from build123d import *

# Parameters (mm, degrees)
BOSS_EXTRUDE1_DEPTH = 4.7625


with BuildPart() as part:
    # Sketch2 → Boss-Extrude1 (new body)
    with BuildSketch(Plane.XY):
        with BuildLine():
            Line((-23, -45.048102255), (-1, -45.048102255))
            ThreePointArc((-1, -45.048102255), (-0.292893219, -45.340995473), (0, -46.048102255))
            Line((0, -46.048102255), (0, -57.748102255))
            Line((0, -57.748102255), (4.7625, -57.748102255))
            Line((4.7625, -57.748102255), (4.7625, -46.048102255))
            ThreePointArc((4.7625, -46.048102255), (5.055393219, -45.340995473), (5.7625, -45.048102255))
            Line((5.7625, -45.048102255), (11.7625, -45.048102255))
            ThreePointArc((11.7625, -45.048102255), (12.469606781, -45.340995473), (12.7625, -46.048102255))
            Line((12.7625, -46.048102255), (12.7625, -69.765561421))
            ThreePointArc((12.7625, -69.765561421), (12.805346982, -70.055144052), (12.9302162, -70.319911199))
            Line((12.9302162, -70.319911199), (68, -153))
            Line((68, -153), (68, -156.7625))
            ThreePointArc((68, -156.7625), (67.707106781, -157.469606781), (67, -157.7625))
            Line((67, -157.7625), (61, -157.7625))
            ThreePointArc((61, -157.7625), (60.292893219, -157.469606781), (60, -156.7625))
            Line((60, -156.7625), (60, -153))
            Line((60, -153), (45.481563848, -153))
            Line((45.481563848, -153), (45.481563848, -156.7625))
            ThreePointArc((45.481563848, -156.7625), (45.188670629, -157.469606781), (44.481563848, -157.7625))
            Line((44.481563848, -157.7625), (38.481563848, -157.7625))
            ThreePointArc((38.481563848, -157.7625), (37.774457067, -157.469606781), (37.481563848, -156.7625))
            Line((37.481563848, -156.7625), (37.481563848, -153))
            Line((37.481563848, -153), (13.059329161, -116.333203921))
            ThreePointArc((13.059329161, -116.333203921), (12.699088908, -116.005978468), (12.227045361, -115.8875537))
            Line((12.227045361, -115.8875537), (-36.227045361, -115.8875537))
            ThreePointArc((-36.227045361, -115.8875537), (-36.699088908, -116.005978468), (-37.059329161, -116.333203921))
            Line((-37.059329161, -116.333203921), (-61.481563848, -153))
            Line((-61.481563848, -153), (-61.481563848, -156.7625))
            ThreePointArc((-61.481563848, -156.7625), (-61.774457067, -157.469606781), (-62.481563848, -157.7625))
            Line((-62.481563848, -157.7625), (-68.481563848, -157.7625))
            ThreePointArc((-68.481563848, -157.7625), (-69.188670629, -157.469606781), (-69.481563848, -156.7625))
            Line((-69.481563848, -156.7625), (-69.481563848, -153))
            Line((-69.481563848, -153), (-84, -153))
            Line((-84, -153), (-84, -156.7625))
            ThreePointArc((-84, -156.7625), (-84.292893219, -157.469606781), (-85, -157.7625))
            Line((-85, -157.7625), (-91, -157.7625))
            ThreePointArc((-91, -157.7625), (-91.707106781, -157.469606781), (-92, -156.7625))
            Line((-92, -156.7625), (-92, -153))
            Line((-92, -153), (-36.9302162, -70.319911199))
            ThreePointArc((-36.9302162, -70.319911199), (-36.805346982, -70.055144052), (-36.7625, -69.765561421))
            Line((-36.7625, -69.765561421), (-36.7625, -46.048102255))
            ThreePointArc((-36.7625, -46.048102255), (-36.469606781, -45.340995473), (-35.7625, -45.048102255))
            Line((-35.7625, -45.048102255), (-29.7625, -45.048102255))
            ThreePointArc((-29.7625, -45.048102255), (-29.055393219, -45.340995473), (-28.7625, -46.048102255))
            Line((-28.7625, -46.048102255), (-28.7625, -57.748102255))
            Line((-28.7625, -57.748102255), (-24, -57.748102255))
            Line((-24, -57.748102255), (-24, -46.048102255))
            ThreePointArc((-24, -46.048102255), (-23.707106781, -45.340995473), (-23, -45.048102255))
        make_face()
    extrude(amount=BOSS_EXTRUDE1_DEPTH)


solid = part.part
Here's how the part is built. I have some questions about the finished solid (model axes, mm). A direction names the side the tool comes from. Give positions to 0.01 mm unless a question says otherwise; leave off trailing zeros. Order: outer loops, then holes, each group sorted by start corner. A loop starts at its lowest first (then second) coordinate and runs counter-clockwise, first axis right, second up. Notation, with made-up numbers: M 12,-26 L 40,-26 A19 cw 40,-12 Z; hole C -40,67.5 d4. An arc over 180 degrees is marked long. Answer as a JSON object with one key per item and string values. Group by question number.
1) Please list where these lines run through material, in increasing order: L1, parallel to X at y = -123.5, z = 0.9; L2, parallel to X at y = -141.5, z = 2.1; L3, parallel to Y at x = -20.5, z = 2.2. Write a range as [from, to].
2) Suppose I cut it at B-B, the plane x = -8. Write out the boundary of the cut face in (y, z).
3) On a 3-axis mill with a long thin cutter (end or side, diameter ignored), from which of +Z, -Z, +X, -X, +Y, -Y can I reach the whole of each face in a straight line? I mean faces 1 (the flat face through (-84, -155, 2)), 2 (the flat face through (0, -52, 2)), 3 (the flat face through (-36.762, -58, 2)). Say none if no direction works.
4) Suppose I cut it at C-C, the plane y = -106. Write out the boundary of the cut face in (x, z), plus the area to 3 significant figures.
5) Suppose I cut it at A-A, the plane y = -123. Write out the boundary of the cut face in (x, z).
6) I'm going to push flat-ended pins straight in: pin 1 Ø1.4 at (y, z) = (-50, 2.5) entering from +X; pin 2 Ø1.5 at (x, z) = (-55, 2.5) entering from -Y; pin 3 Ø1.4 at (x, z) = (-75.5, 2.5) entering from -Y. Where does each tip first touch, or does it pass through?
7) We'd pull the mould along X, two halves only. Please class faces 4 (the flat face through (-26, -57.748, 2)), 5 (the flat face through (-92, -155, 2)), 6 (the flat face through (-12, -45.048, 2)): pulls with the +X half, pulls with the -X half, needs draft (parallel to the pull), parting line crosses it, or undercut.
Results found:
{
 "1": {"L1": "[-72.35, -41.83], [17.83, 48.35]", "L2": "[-84.34, -53.82], [29.82, 60.34]", "L3": "[-115.89, -45.05]"},
 "2": {"outline": "M -115.89,0 L -45.05,0 L -45.05,4.76 L -115.89,4.76 Z"},
 "3": {"face 1": "+Z, -Z, -Y", "face 2": "+Z, -Z, +Y", "face 3": "+Z, -Z, -X, +Y"},
 "4": {"outline": "M -60.7,0 L 36.7,0 L 36.7,4.76 L -60.7,4.76 Z", "area": "464 mm²"},
 "5": {"outline": "M -72.02,0 L -41.5,0 L -41.5,4.76 L -72.02,4.76 Z; M 17.5,0 L 48.02,0 L 48.02,4.76 L 17.5,4.76 Z"},
 "6": {"pin 1": "x = 12.76", "pin 2": "y = -144.39", "pin 3": "y = -153"},
 "7": {"face 4": "undercut", "face 5": "pulls with the -X half", "face 6": "needs draft"}
}
